Geometry check sheet. Reference: the model listing, model coordinates, mm. A direction names the side the tool comes from. Round coordinates to 2 decimals unless told otherwise and drop trailing zeros. Order: outer loops, then holes, each group sorted by start corner. A loop starts at its lowest first (then second) coordinate and runs counter-clockwise, first axis right, second up.
(1) Sectioned sample at D-D (z = -0.6). Record the boundary of the cut face in (x, y).
(2) Sectioned sample at A-A (y = 5.85). Record the boundary of the cut face in (x, z).
(3) Sectioned sample at C-C (x = 0). Record the boundary of the cut face in (y, z).
(4) Set-up check for faces 4 (the face through (0, 0, 0)), 5 (the face through (-5, 17, -3)), 6 (the face through (-12.096, 26.165, -0.43)), 7 (the face through (-10.05, 5.91, -3.47)): record each of +Z, -Z, +X, -X, +Y, -Y from which the full face is reachable in a straight line by a thin tool's end or side.
(5) Material ranges on line 1 along X through (y, z) = (28.85, -4.1); line 2 along Y through (x, z) = (-11.5, -3.85); line 3 along Y through (x, z) = (11, -2.75), recorded low to high.
(6) Release check for a two-part mould opening along Y. For faces 1 (the face through (-15, 14, -2)), 2 (the face through (12.95, 5.91, -3.47)), 3 (the face through (-14.43, 31.4, -2.04)) record: +Y half, -Y half, draft (parallel to the pull), parting line (faces both ways), or undercut.
(7) Go/stop test with flat-tipped pins: pin 1 (5 mm diameter, centred on x = -11.5, y = 5.85, fed in from +Z); pin 2 (0.8 mm diameter, centred on x = 6, z = 0.5, fed in from -Y); pin 3 (5 mm diameter, centred on x = 0, y = 17.35, fed in from +Z); pin 4 (4.5 mm diameter, centred on x = 1, y = -1, fed in from +Z). Record where each tip stops, or that it passes through.
(8) Sectioned sample at B-B (x = -11.5). Record the boundary of the cut face in (y, z), plus the area to 3 significant figures.
from build123d import *

# Parameters (mm, degrees)
BODY_DEPTH               = 30
FIXTURE_M2_5_D           = 2.9
FIXTURE_M2_5_DEPTH       = 6
FIXTURE_M2_5_CBORE_D     = 5.5
FIXTURE_M2_5_CBORE_DEPTH = 2.9
FIXTURE_M2_5_TIP         = 0.871247898
SKETCH_5_R               = 4
CUT_EXTRUDE_1_DEPTH      = 6
SKETCH_6_R               = 11
CUT_EXTRUDE_2_DEPTH      = 2
FILLET_1_R               = 2


with BuildPart() as part:
    # Эскиз1 → Body (new body)
    with BuildSketch(Plane.ZY.offset(15)):
        Polygon((1, 2.7), (1, 32), (-5, 32), (-5, -3), (0, -3), (0, 2.7), align=None)
    extrude(amount=-BODY_DEPTH)

    # Fixture M2.5
    with Locations(Plane(origin=(-11.5, 28.85, 1), x_dir=(1, 0, 0), z_dir=(0, 0, 1))):
        with Locations((0, 0), (23, 0), (23, -23), (0, -23)):
            CounterBoreHole(FIXTURE_M2_5_D / 2, FIXTURE_M2_5_CBORE_D / 2, FIXTURE_M2_5_CBORE_DEPTH, depth=FIXTURE_M2_5_DEPTH)
            with Locations((0, 0, -(FIXTURE_M2_5_DEPTH + FIXTURE_M2_5_TIP / 2))):  # 118° drill point
                Cone(0, FIXTURE_M2_5_D / 2, FIXTURE_M2_5_TIP, mode=Mode.SUBTRACT)

    # Эскиз5 → Вырез-Вытянуть1 (cut)
    with BuildSketch(Plane.XY.offset(1)):
        with Locations((0, 17.35)):
            Circle(SKETCH_5_R)
    extrude(amount=-CUT_EXTRUDE_1_DEPTH, mode=Mode.SUBTRACT)

    # Эскиз6 → Вырез-Вытянуть2 (cut)
    with BuildSketch(Plane(origin=(0, 0, -5), x_dir=(-1, 0, 0), z_dir=(0, 0, -1))):
        with Locations(Location((0, 17.35, 0), (0, 0, 90))):
            Circle(SKETCH_6_R)
    extrude(amount=-CUT_EXTRUDE_2_DEPTH, mode=Mode.SUBTRACT)

    # Скругление1
    fillet_1_edges = [part.edges().sort_by_distance(p)[0] for p in [
        (15, 32, -2),
        (-15, 32, -2),
    ]]
    fillet(fillet_1_edges, radius=FILLET_1_R)


solid = part.part
Answer below:
1. outline: (-15, -3) - (15, -3) - (15, 30) arc R2 ccw to (13, 32) - (-13, 32) arc R2 ccw to (-15, 30) - close; hole circle Ø5.5 at (-11.5, 5.85); hole circle Ø5.5 at (-11.5, 28.85); hole circle Ø8 at (0, 17.35); hole circle Ø5.5 at (11.5, 5.85); hole circle Ø5.5 at (11.5, 28.85)
2. outline: (-15, -5) - (-12.95, -5) - (-12.95, -1.9) - (-14.25, -1.9) - (-14.25, 1) - (-15, 1) - close; (-10.05, -5) - (10.05, -5) - (10.05, -1.9) - (8.75, -1.9) - (8.75, 1) - (-8.75, 1) - (-8.75, -1.9) - (-10.05, -1.9) - close; (12.95, -5) - (15, -5) - (15, 1) - (14.25, 1) - (14.25, -1.9) - (12.95, -1.9) - close
3. outline: (-3, -5) - (6.35, -5) - (6.35, -3) - (13.35, -3) - (13.35, 1) - (2.7, 1) - (2.7, 0) - (-3, 0) - close; (21.35, -3) - (28.35, -3) - (28.35, -5) - (32, -5) - (32, 1) - (21.35, 1) - close
4. face 4: +Z, +X, -X, -Y
4. face 5: -Z
4. face 6: +Z
4. face 7: +Z, -Z
5. line 1: x = -15 to -12.95, -10.05 to 10.05, 12.95 to 15
5. line 2: y = -3 to 4.4, 7.3 to 27.4, 30.3 to 32
5. line 3: y = -3 to 4.49, 7.21 to 27.49, 30.21 to 32
6. face 1: draft
6. face 2: undercut
6. face 3: +Y half
7. pin 1: stops at z = -1.9
7. pin 2: stops at y = 2.7
7. pin 3: passes through
7. pin 4: stops at z = 0
8. outline: (-3, -5) - (4.4, -5) - (4.4, -1.9) - (3.1, -1.9) - (3.1, 1) - (2.7, 1) - (2.7, 0) - (-3, 0) - close; (7.3, -5) - (27.4, -5) - (27.4, -1.9) - (26.1, -1.9) - (26.1, 1) - (8.6, 1) - (8.6, -1.9) - (7.3, -1.9) - close; (30.3, -5) - (32, -5) - (32, 1) - (31.6, 1) - (31.6, -1.9) - (30.3, -1.9) - close
8. area: 154 mm2
